Verification items for the finished model (mm, model axes). A direction names the side the tool comes from. Give positions to 0.01 mm unless a question says otherwise; leave off trailing zeros. Loops run counter-clockwise (first coordinate to the right, second up) from the corner with the lowest first, then second, coordinate; pieces in that order, holes last. Notation, with made-up numbers: (54, 69) -> (111, 69) arc R20 ccw to (111, 78) -> close; hole circle Ø8 at (34, -5). An arc over 180 degrees is marked (long way). Answer in a Markdown table with one row per item. Add a question column.
Q1. Section check C-C on y = 8. Enter the section's corners in (x, z).
Q2. Set-up check for faces 5 (the face through (-91.493, -1.127, 36.412)), 6 (the face through (244.844, -9, 35)), 7 (the face through (-3, 10, 86.614)): record each of +Z, -Z, +X, -X, +Y, -Y from which the full face is reachable in a straight line by a thin tool's end or side.
Q3. Section check B-B on x = -168.5. Enter the section's corners in (y, z), and give its area (3 significant figures).
Q4. Material ranges on probe 1 along X at (y, z) = (-5.5, 24.5); probe 2 along Y at (x, z) = (22, -1.5); probe 3 along X at (y, z) = (-1.5, 70.5), recorded low to high.
Q5. Gauge pin test, flat ends, axial feed: P1, Ø6, axis at x = -181.37, z = 58.11, coming from the -Y side; P2, Ø1, axis at x = -123, z = 4, coming from the +Y side; P3, Ø3.5, axis at x = -243.5, y = -7, coming from the +Z side. Record the tip position at first contact, or that the pin passes through.
Q6. Section check A-A on x = -17. Enter the section's corners in (y, z), and give its area (3 significant figures).
Q7. Release check for a two-part mould opening along X. For faces 1 (the face through (-244.844, -10, 36)), 2 (the face through (247.13, -10, 35)), 3 (the face through (0, -1, -12.7)), 4 (the face through (17.497, -1.127, 35.576)) record: pulls with the +X half, pulls with the -X half, needs draft (parallel to the pull), parting line crosses it, or undercut.
```python
from build123d import *

# Parameters (mm, degrees)
SKETCH1_W                    = 489.688000048
SKETCH1_H                    = 177.8
BASE_FLANGE1_DEPTH           = 2.286
EDGE_FLANGE1_STRIP_W         = 13.864
EDGE_FLANGE1_STRIP_H         = 2.286
EDGE_FLANGE1_STRIP_CUT_DEPTH = 489.688000048
EDGE_FLANGE1_DEPTH           = 489.688000048
EDGE_FLANGE2_STRIP_W         = 13.864
EDGE_FLANGE2_STRIP_H         = 2.286
EDGE_FLANGE2_STRIP_CUT_DEPTH = 173.154
EDGE_FLANGE2_DEPTH           = 173.154
EDGE_FLANGE3_STRIP_W         = 13.864
EDGE_FLANGE3_STRIP_H         = 2.286
EDGE_FLANGE3_STRIP_CUT_DEPTH = 173.154
EDGE_FLANGE3_DEPTH           = 173.154
SKETCH15_R                   = 3.15
CUT_EXTRUDE1_DEPTH           = 6.35
SKETCH33_W                   = 491.974000048
SKETCH33_H                   = 152.4
CUT_EXTRUDE5_DEPTH           = 264.323659043
SKETCH40_R                   = 2.413
CUT_EXTRUDE10_DEPTH          = 501.304436542
SKETCH42_R                   = 2.4
CUT_EXTRUDE11_DEPTH          = 264.323659043


# Sheet-metal steps are written as plain solids
with BuildPart() as part:
    # Sketch1 → Base-Flange1 (new body)
    with BuildSketch(Plane(origin=(0, 0, 0), x_dir=(1, 0, 0), z_dir=(0, 1, 0))):
        Rectangle(SKETCH1_W, SKETCH1_H)
    extrude(amount=-BASE_FLANGE1_DEPTH)

    # Edge-Flange1 strip (across the edge) → Edge-Flange1 strip cut (cut)
    with BuildSketch(Plane(origin=(-244.844000024, 0, 88.9), x_dir=(0, 0, -1), z_dir=(1, 0, 0))):
        with Locations((-2.286, -1.143)):
            Rectangle(EDGE_FLANGE1_STRIP_W, EDGE_FLANGE1_STRIP_H)
    extrude(amount=EDGE_FLANGE1_STRIP_CUT_DEPTH, mode=Mode.SUBTRACT)

    # Edge-Flange1 section (across the edge) → Edge-Flange1 (add)
    with BuildSketch(Plane(origin=(-244.844000024, 0, 88.9), x_dir=(0, 0, -1), z_dir=(1, 0, 0))):
        with BuildLine():
            Line((0, 2.36), (0, 16.764))
            Line((0, 16.764), (2.286, 16.764))
            Line((2.286, 16.764), (2.286, 2.36))
            ThreePointArc((2.286, 2.36), (2.977227996, 0.691227996), (4.646, 0))
            Line((4.646, 0), (4.646, -2.286))
            ThreePointArc((4.646, -2.286), (1.360781895, -0.925218105), (0, 2.36))
        make_face()
    extrude(amount=EDGE_FLANGE1_DEPTH)

    # Edge-Flange2 strip (across the edge) → Edge-Flange2 strip cut (cut)
    with BuildSketch(Plane(origin=(-244.844000024, -2.286, 84.254), x_dir=(1, 0, 0), z_dir=(0, 0, -1))):
        with Locations((-2.286, -1.143)):
            Rectangle(EDGE_FLANGE2_STRIP_W, EDGE_FLANGE2_STRIP_H)
    extrude(amount=EDGE_FLANGE2_STRIP_CUT_DEPTH, mode=Mode.SUBTRACT)

    # Edge-Flange2 section (across the edge) → Edge-Flange2 (add)
    with BuildSketch(Plane(origin=(-244.844000024, -2.286, 84.254), x_dir=(1, 0, 0), z_dir=(0, 0, -1))):
        with BuildLine():
            Line((0, 2.36), (0, 16.764))
            Line((0, 16.764), (2.286, 16.764))
            Line((2.286, 16.764), (2.286, 2.36))
            ThreePointArc((2.286, 2.36), (2.977227996, 0.691227996), (4.646, 0))
            Line((4.646, 0), (4.646, -2.286))
            ThreePointArc((4.646, -2.286), (1.360781895, -0.925218105), (0, 2.36))
        make_face()
    extrude(amount=EDGE_FLANGE2_DEPTH)

    # Edge-Flange3 strip (across the edge) → Edge-Flange3 strip cut (cut)
    with BuildSketch(Plane(origin=(244.844000024, -2.286, -88.9), x_dir=(-1, 0, 0), z_dir=(0, 0, 1))):
        with Locations((-4.572, -1.143)):
            Rectangle(EDGE_FLANGE3_STRIP_W, EDGE_FLANGE3_STRIP_H)
    extrude(amount=EDGE_FLANGE3_STRIP_CUT_DEPTH, mode=Mode.SUBTRACT)

    # Edge-Flange3 section (across the edge) → Edge-Flange3 (add)
    with BuildSketch(Plane(origin=(244.844000024, -2.286, -88.9), x_dir=(-1, 0, 0), z_dir=(0, 0, 1))):
        with BuildLine():
            Line((-2.286, 2.36), (-2.286, 16.764))
            Line((-2.286, 16.764), (0, 16.764))
            Line((0, 16.764), (0, 2.36))
            ThreePointArc((0, 2.36), (0.691227996, 0.691227996), (2.36, 0))
            Line((2.36, 0), (2.36, -2.286))
            ThreePointArc((2.36, -2.286), (-0.925218105, -0.925218105), (-2.286, 2.36))
        make_face()
    extrude(amount=EDGE_FLANGE3_DEPTH)

    # Sketch15 → Cut-Extrude1 (cut)
    with BuildSketch(Plane(origin=(0, 0, 0), x_dir=(1, 0, 0), z_dir=(0, 1, 0))):
        with Locations(Location((-92.248000024, -1.994, 0), (0, 0, 270))):
            Circle(SKETCH15_R)
        with Locations(Location((-92.248000024, -69.994, 0), (0, 0, 270))):
            Circle(SKETCH15_R)
        with Locations(Location((18.251999976, -69.994, 0), (0, 0, 270))):
            Circle(SKETCH15_R)
        with Locations(Location((18.251999976, -1.994, 0), (0, 0, 270))):
            Circle(SKETCH15_R)
        with BuildLine():
            Line((-1.498000024, -54.994), (-72.498000024, -54.994))
            ThreePointArc((-72.498000024, -54.994), (-91.498000024, -35.994), (-72.498000024, -16.994))
            Line((-72.498000024, -16.994), (-1.498000024, -16.994))
            ThreePointArc((-1.498000024, -16.994), (17.501999976, -35.994), (-1.498000024, -54.994))
        make_face()
    extrude(amount=-CUT_EXTRUDE1_DEPTH, mode=Mode.SUBTRACT)

    # Sketch33 → Cut-Extrude5 (cut, through all)
    with BuildSketch(Plane(origin=(0, 0, 0), x_dir=(1, 0, 0), z_dir=(0, 1, 0))):
        with Locations((1.143, 88.9)):
            Rectangle(SKETCH33_W, SKETCH33_H)
    extrude(amount=-CUT_EXTRUDE5_DEPTH, mode=Mode.SUBTRACT)

    # Sketch40 → Cut-Extrude10 (cut, through all)
    with BuildSketch(Plane.ZY.offset(244.844000024)):
        with Locations(Location((77.904, -12.7, 0), (0, 0, 270))):
            Circle(SKETCH40_R)
        with Locations(Location((63.6165, -12.7, 0), (0, 0, 270))):
            Circle(SKETCH40_R)
        with Locations(Location((49.329, -12.7, 0), (0, 0, 270))):
            Circle(SKETCH40_R)
        with Locations(Location((35.0415, -12.7, 0), (0, 0, 270))):
            Circle(SKETCH40_R)
        with Locations(Location((20.754, -12.7, 0), (0, 0, 270))):
            Circle(SKETCH40_R)
        with Locations(Location((6.4665, -12.7, 0), (0, 0, 270))):
            Circle(SKETCH40_R)
        with Locations(Location((-7.821, -12.7, 0), (0, 0, 270))):
            Circle(SKETCH40_R)
    extrude(amount=-CUT_EXTRUDE10_DEPTH, mode=Mode.SUBTRACT)

    # Sketch42 → Cut-Extrude11 (cut, through all)
    with BuildSketch(Plane(origin=(0, 0, 0), x_dir=(1, 0, 0), z_dir=(0, 1, 0))):
        with Locations(Location((-220.419354597, -14.058539081, 0), (0, 0, 270))):
            Circle(SKETCH42_R)
        with Locations(Location((-181.369354597, -14.058539081, 0), (0, 0, 270))):
            Circle(SKETCH42_R)
        with Locations(Location((-181.369354597, -58.108539081, 0), (0, 0, 270))):
            Circle(SKETCH42_R)
        with Locations(Location((-220.419354597, -58.108539081, 0), (0, 0, 270))):
            Circle(SKETCH42_R)
    extrude(amount=-CUT_EXTRUDE11_DEPTH, mode=Mode.SUBTRACT)


solid = part.part
```
Taken from the geometry:
| question | item | result |
|---|---|---|
| 1 | outline | (-244.84, 86.61) -> (244.84, 86.61) -> (244.84, 88.9) -> (-244.84, 88.9) -> close |
| 2 | face 5 | +Y, -Y |
| 2 | face 6 | +Z, -Z, -Y |
| 2 | face 7 | -Z, +X, -X, +Y |
| 3 | outline | (-2.29, -12.7) -> (0, -12.7) -> (0, 84.25) arc R2.36 cw to (2.36, 86.61) -> (16.76, 86.61) -> (16.76, 88.9) -> (2.36, 88.9) arc R4.65 ccw to (-2.29, 84.25) -> close |
| 3 | area | 267 mm² |
| 4 | probe 1 | x = -244.84 to -242.56, 244.84 to 247.13 |
| 4 | probe 2 | y = -2.29 to 0 |
| 4 | probe 3 | x = -243.62 to -95.36, -89.14 to 15.14, 21.36 to 245.9 |
| 5 | P1 | stops at y = -2.29 |
| 5 | P2 | stops at y = 0 |
| 5 | P3 | stops at z = 84.25 |
| 6 | outline | (-2.29, -12.7) -> (0, -12.7) -> (0, 16.99) -> (-2.29, 16.99) -> close; (-2.29, 54.99) -> (0, 54.99) -> (0, 84.25) arc R2.36 cw to (2.36, 86.61) -> (16.76, 86.61) -> (16.76, 88.9) -> (2.36, 88.9) arc R4.65 ccw to (-2.29, 84.25) -> close |
| 6 | area | 180 mm² |
| 7 | face 1 | pulls with the -X half |
| 7 | face 2 | pulls with the +X half |
| 7 | face 3 | needs draft |
| 7 | face 4 | undercut |
